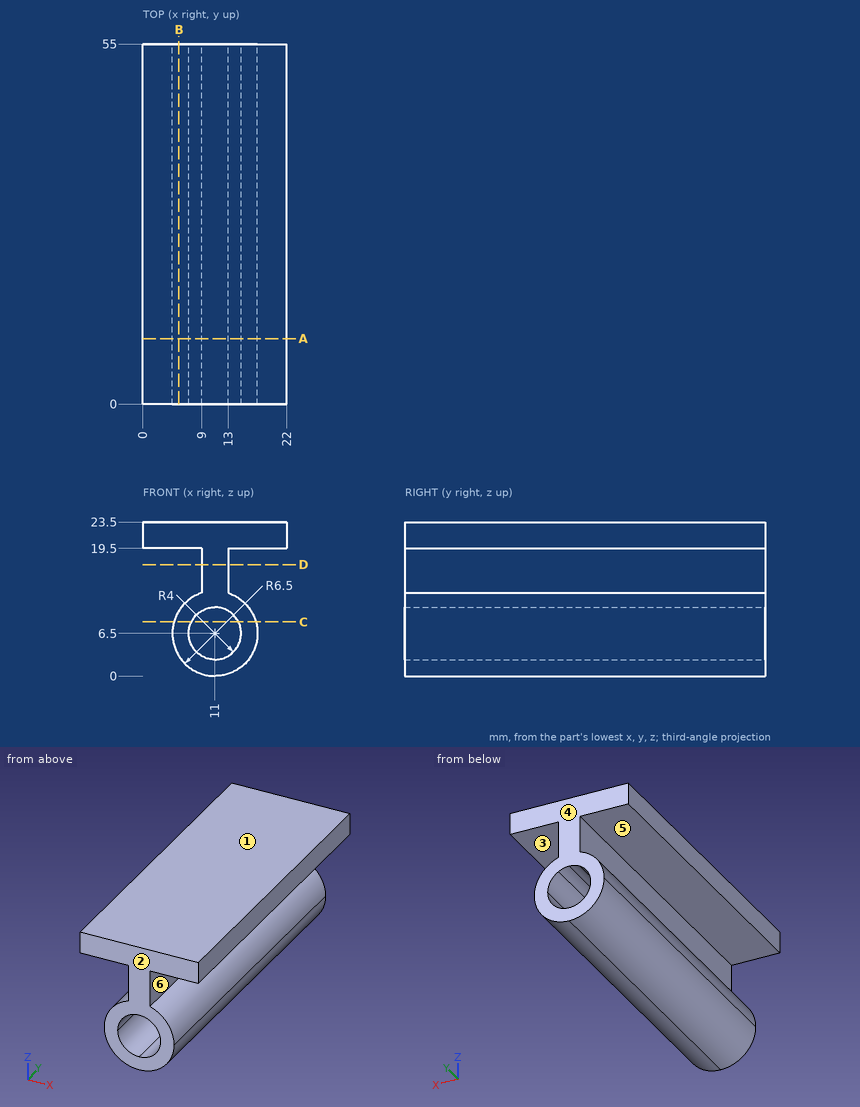
Job drawing, mm, ordinate dimensions from the low corner. One solid piece. A direction names the side the tool comes from. Give positions to 0.01 mm unless a question says otherwise; leave off trailing zeros. Loops run counter-clockwise (first coordinate to the right, second up) from the corner with the lowest first, then second, coordinate; pieces in that order, holes last. Notation, with made-up numbers: M 73,-8.5 L 115,-8.5 A22 cw 115,-1.5 Z; hole C 32,45 d6. An arc over 180 degrees is marked long. Put each result on its own line as item: value. Start each with the question number.
1) Probe probe 1 along Z at (x, y) = (8.25, 36); probe 2 along Z at (x, y) = (13.5, 8.5); probe 3 along Z at (x, y) = (3.5, 22.5). List the from-to ranges inside material, lowest first.
2) Saw through at B-B (x = 5.5). List the corners of the cut face in (y, z).
3) Saw through at D-D (z = 17). List the corners of the cut face in (x, y).
4) Saw through at A-A (y = 10). List the corners of the cut face in (x, z), then the cut area to 3 significant figures.
5) Pull direction Z, two halves, no side cores. Call the marked faces 1, 2 and 3: +Z half, -Z half, draft (parallel to the pull), parting line (faces both ways), or undercut.
6) 3-axis set-ups, long thin cutter, end or side, ignore diameter. For the marked faces 4, 5 and 6: which of +Z, -Z, +X, -X, +Y, -Y reach the whole face in a straight line?
7) Saw through at C-C (z = 8.25). List the corners of the cut face in (x, y), then the cut area to 3 significant figures.
8) Flat gauge pins, fed straight in: pin 1 (5 mm diameter, centred on y = 23.5, z = 15.5, fed in from -X); pin 2 (8 mm diameter, centred on y = 12.5, z = 21, fed in from -X); pin 3 (4.5 mm diameter, centred on x = 16, y = 14.5, fed in from -Z); pin 4 (3 mm diameter, centred on y = 42, z = 14, fed in from -X). Where does each tip first touch, or does it go through?
Numbers:
1. probe 1: 0.61 to 3.6, 9.4 to 12.39, 19.5 to 23.5
1. probe 2: 0.5 to 3.38, 9.62 to 12.5, 19.5 to 23.5
1. probe 3: 19.5 to 23.5
2. outline: M 0,3.04 L 55,3.04 L 55,9.96 L 0,9.96 Z; M 0,19.5 L 55,19.5 L 55,23.5 L 0,23.5 Z
3. outline: M 9,0 L 13,0 L 13,55 L 9,55 Z
4. outline: M 0,19.5 L 9,19.5 L 9,12.68 A6.5 ccw long 13,12.68 L 13,19.5 L 22,19.5 L 22,23.5 L 0,23.5 Z; hole C 11,6.5 d8
4. area: 197 mm^2
5. face 1: +Z half
5. face 2: draft
5. face 3: undercut
6. face 4: +Z, -Z, +X, -X, +Y
6. face 5: -X, +Y, -Y
6. face 6: +X, +Y, -Y
7. outline: M 4.74,0 L 7.4,0 L 7.4,55 L 4.74,55 Z; M 14.6,0 L 17.26,0 L 17.26,55 L 14.6,55 Z
7. area: 293 mm^2
8. pin 1: x = 9
8. pin 2: x = 0
8. pin 3: z = 0.61
8. pin 4: x = 8.5
